Source: CAD feature listing. Evaluate the final solid. Frame: model axes, mm. Give positions to 0.01 mm unless a question says otherwise; leave off trailing zeros. Answer as a JSON object with one key per item and string values. Group by question number.
from build123d import *

# Parameters (mm, degrees)
SKETCH1_R               = 2.6035
BOSS_EXTRUDE1_DEPTH     = 539.0896
CUT_EXTRUDE2_DEPTH      = 13.7
CUT_EXTRUDE2_DEPTH_BACK = 13.7


with BuildPart() as part:
    # Sketch1 → Boss-Extrude1 (new body, symmetric)
    with BuildSketch(Plane(origin=(0, 0, -450.85), x_dir=(-1, 0, 0), z_dir=(0, 0, -1))):
        with BuildLine():
            Line((12.7, -9.5504), (12.7, -6.3330836))
            ThreePointArc((12.7, -6.3330836), (12.192, -5.8250836), (12.7, -5.3170836))
            Line((12.7, -5.3170836), (12.7, -4.3434))
            ThreePointArc((12.7, -4.3434), (11.5951, -3.2385), (10.4902, -4.3434))
            Line((10.4902, -4.3434), (10.4902, -6.474794456))
            ThreePointArc((10.4902, -6.474794456), (9.863006367, -7.413456061), (8.75577951, -7.193214945))
            Line((8.75577951, -7.193214945), (5.42573597, -3.863171405))
            ThreePointArc((5.42573597, -3.863171405), (4.737482484, -2.833127272), (4.4958, -1.618107374))
            Line((4.4958, -1.618107374), (4.4958, 1.618107374))
            ThreePointArc((4.4958, 1.618107374), (4.737482484, 2.833127272), (5.42573597, 3.863171405))
            Line((5.42573597, 3.863171405), (8.75577951, 7.193214945))
            ThreePointArc((8.75577951, 7.193214945), (9.863006367, 7.413456061), (10.4902, 6.474794456))
            Line((10.4902, 6.474794456), (10.4902, 4.343399971))
            ThreePointArc((10.4902, 4.343399971), (11.5951, 3.238499971), (12.7, 4.343399971))
            Line((12.7, 4.343399971), (12.7, 5.3170836))
            ThreePointArc((12.7, 5.3170836), (12.192, 5.8250836), (12.7, 6.3330836))
            Line((12.7, 6.3330836), (12.7, 9.5504))
            ThreePointArc((12.7, 9.5504), (12.192000006, 10.058323491), (12.699846982, 10.566399977))
            ThreePointArc((12.699846982, 10.566399977), (12.082522516, 12.082522516), (10.566399977, 12.699846982))
            ThreePointArc((10.566399977, 12.699846982), (10.058323491, 12.192000006), (9.5504, 12.7))
            Line((9.5504, 12.7), (6.3330836, 12.7))
            ThreePointArc((6.3330836, 12.7), (5.8250836, 12.192), (5.3170836, 12.7))
            Line((5.3170836, 12.7), (4.3434, 12.7))
            ThreePointArc((4.3434, 12.7), (3.2385, 11.5951), (4.3434, 10.4902))
            Line((4.3434, 10.4902), (6.474794456, 10.4902))
            ThreePointArc((6.474794456, 10.4902), (7.413456061, 9.863006367), (7.193214945, 8.75577951))
            Line((7.193214945, 8.75577951), (3.863171405, 5.42573597))
            ThreePointArc((3.863171405, 5.42573597), (2.833127272, 4.737482484), (1.618107374, 4.4958))
            Line((1.618107374, 4.4958), (-1.618107374, 4.4958))
            ThreePointArc((-1.618107374, 4.4958), (-2.833127272, 4.737482484), (-3.863171405, 5.42573597))
            Line((-3.863171405, 5.42573597), (-7.193214945, 8.75577951))
            ThreePointArc((-7.193214945, 8.75577951), (-7.413456061, 9.863006367), (-6.474794456, 10.4902))
            Line((-6.474794456, 10.4902), (-4.343399971, 10.4902))
            ThreePointArc((-4.343399971, 10.4902), (-3.238499971, 11.5951), (-4.343399971, 12.7))
            Line((-4.343399971, 12.7), (-5.3170836, 12.7))
            ThreePointArc((-5.3170836, 12.7), (-5.8250836, 12.192), (-6.3330836, 12.7))
            Line((-6.3330836, 12.7), (-9.5504, 12.7))
            ThreePointArc((-9.5504, 12.7), (-10.058323491, 12.192000006), (-10.566399977, 12.699846982))
            ThreePointArc((-10.566399977, 12.699846982), (-12.082522516, 12.082522516), (-12.699846982, 10.566399977))
            ThreePointArc((-12.699846982, 10.566399977), (-12.192000006, 10.058323491), (-12.7, 9.5504))
            Line((-12.7, 9.5504), (-12.7, 6.3330836))
            ThreePointArc((-12.7, 6.3330836), (-12.192, 5.8250836), (-12.7, 5.3170836))
            Line((-12.7, 5.3170836), (-12.7, 4.3434))
            ThreePointArc((-12.7, 4.3434), (-11.5951, 3.2385), (-10.4902, 4.3434))
            Line((-10.4902, 4.3434), (-10.4902, 6.474794456))
            ThreePointArc((-10.4902, 6.474794456), (-9.863006367, 7.413456061), (-8.75577951, 7.193214945))
            Line((-8.75577951, 7.193214945), (-5.42573597, 3.863171405))
            ThreePointArc((-5.42573597, 3.863171405), (-4.737482484, 2.833127272), (-4.4958, 1.618107374))
            Line((-4.4958, 1.618107374), (-4.4958, -1.618107374))
            ThreePointArc((-4.4958, -1.618107374), (-4.737482484, -2.833127272), (-5.42573597, -3.863171405))
            Line((-5.42573597, -3.863171405), (-8.75577951, -7.193214945))
            ThreePointArc((-8.75577951, -7.193214945), (-9.863006367, -7.413456061), (-10.4902, -6.474794456))
            Line((-10.4902, -6.474794456), (-10.4902, -4.343399971))
            ThreePointArc((-10.4902, -4.343399971), (-11.5951, -3.238499971), (-12.7, -4.343399971))
            Line((-12.7, -4.343399971), (-12.7, -5.3170836))
            ThreePointArc((-12.7, -5.3170836), (-12.192, -5.8250836), (-12.7, -6.3330836))
            Line((-12.7, -6.3330836), (-12.7, -9.5504))
            ThreePointArc((-12.7, -9.5504), (-12.192000006, -10.058323491), (-12.699846982, -10.566399977))
            ThreePointArc((-12.699846982, -10.566399977), (-12.082522516, -12.082522516), (-10.566399977, -12.699846982))
            ThreePointArc((-10.566399977, -12.699846982), (-10.058323491, -12.192000006), (-9.5504, -12.7))
            Line((-9.5504, -12.7), (-6.3330836, -12.7))
            ThreePointArc((-6.3330836, -12.7), (-5.8250836, -12.192), (-5.3170836, -12.7))
            Line((-5.3170836, -12.7), (-4.3434, -12.7))
            ThreePointArc((-4.3434, -12.7), (-3.2385, -11.5951), (-4.3434, -10.4902))
            Line((-4.3434, -10.4902), (-6.474794456, -10.4902))
            ThreePointArc((-6.474794456, -10.4902), (-7.413456061, -9.863006367), (-7.193214945, -8.75577951))
            Line((-7.193214945, -8.75577951), (-3.863171405, -5.42573597))
            ThreePointArc((-3.863171405, -5.42573597), (-2.833127272, -4.737482484), (-1.618107374, -4.4958))
            Line((-1.618107374, -4.4958), (1.618107374, -4.4958))
            ThreePointArc((1.618107374, -4.4958), (2.833127272, -4.737482484), (3.863171405, -5.42573597))
            Line((3.863171405, -5.42573597), (7.193214945, -8.75577951))
            ThreePointArc((7.193214945, -8.75577951), (7.413456061, -9.863006367), (6.474794456, -10.4902))
            Line((6.474794456, -10.4902), (4.343399971, -10.4902))
            ThreePointArc((4.343399971, -10.4902), (3.238499971, -11.5951), (4.343399971, -12.7))
            Line((4.343399971, -12.7), (5.3170836, -12.7))
            ThreePointArc((5.3170836, -12.7), (5.8250836, -12.192), (6.3330836, -12.7))
            Line((6.3330836, -12.7), (9.5504, -12.7))
            ThreePointArc((9.5504, -12.7), (10.058323491, -12.192000006), (10.566399977, -12.699846982))
            ThreePointArc((10.566399977, -12.699846982), (12.082522516, -12.082522516), (12.699846982, -10.566399977))
            ThreePointArc((12.699846982, -10.566399977), (12.192000006, -10.058323491), (12.7, -9.5504))
        make_face()
        Circle(SKETCH1_R, mode=Mode.SUBTRACT)
    extrude(amount=BOSS_EXTRUDE1_DEPTH, both=True)

    # Sketch2 → Cut-Extrude2 (cut, two sides)
    with BuildSketch(Plane(origin=(0, 0, 0), x_dir=(0, 0, -1), z_dir=(1, 0, 0))) as cut_extrude2_sk:
        Polygon((-79.030508577, 8.745212893), (-88.2396, 12.699846982), (-101.048292807, 21.699279404), (-97.311113584, -6.062623399), (-88.2396, -12.699846982), align=None)
        Polygon((990.442416852, 50.12885935), (974.65896, 12.699846982), (952.537969595, -34.847055216), (990.442416852, -34.847055216), align=None)
    extrude(amount=CUT_EXTRUDE2_DEPTH, mode=Mode.SUBTRACT)
    extrude(cut_extrude2_sk.sketch, amount=-CUT_EXTRUDE2_DEPTH_BACK, mode=Mode.SUBTRACT)


solid = part.part
(1) Mould query, pull axis Y, two halves, no side actions, for faces 1 (the face through (-2.64, -2.13, 83.7)), 2 (the face through (3, 0.178, -968.833)). Classes: pulls with the +Y half, pulls with the -Y half, needs draft (parallel to the pull), parting line crosses it, or undercut.
(2) First-contact query: pin 1 (3 mm diameter, centred on x = -2.5, y = -5, fed in from -Z); pin 2 (1 mm diameter, centred on y = -3.5, z = -461.5, fed in from -X); pin 3 (8.5 mm diameter, centred on x = 0, y = 0, fed in from +Z); pin 4 (5 mm diameter, centred on x = -0.5, y = -8, fed in from -Z). Flat tips, straight axial feed; report the tip coordinate or a pass-through.
(3) Material intervals for line 1 (X direction, y = -5.5, z = -696.5); line 2 (Y direction, x = -5, z = -588.5); line 3 (X direction, y = 0, z = -378), sorted ascending. Write a range as from..to.
Result:
{
 "1": {"face 1": "undercut", "face 2": "pulls with the -Y half"},
 "2": {"pin 1": "z = -967.12", "pin 2": "x = -12.65", "pin 3": "z = 84.61", "pin 4": "through"},
 "3": {"line 1": "-12.31..-10.49, -7.06..-3.94, 3.94..7.06, 10.49..12.31", "line 2": "-12.7..-10.49, -6.56..-3.33, 3.33..6.56, 10.49..12.7", "line 3": "-4.5..-2.6, 2.6..4.5"}
}
